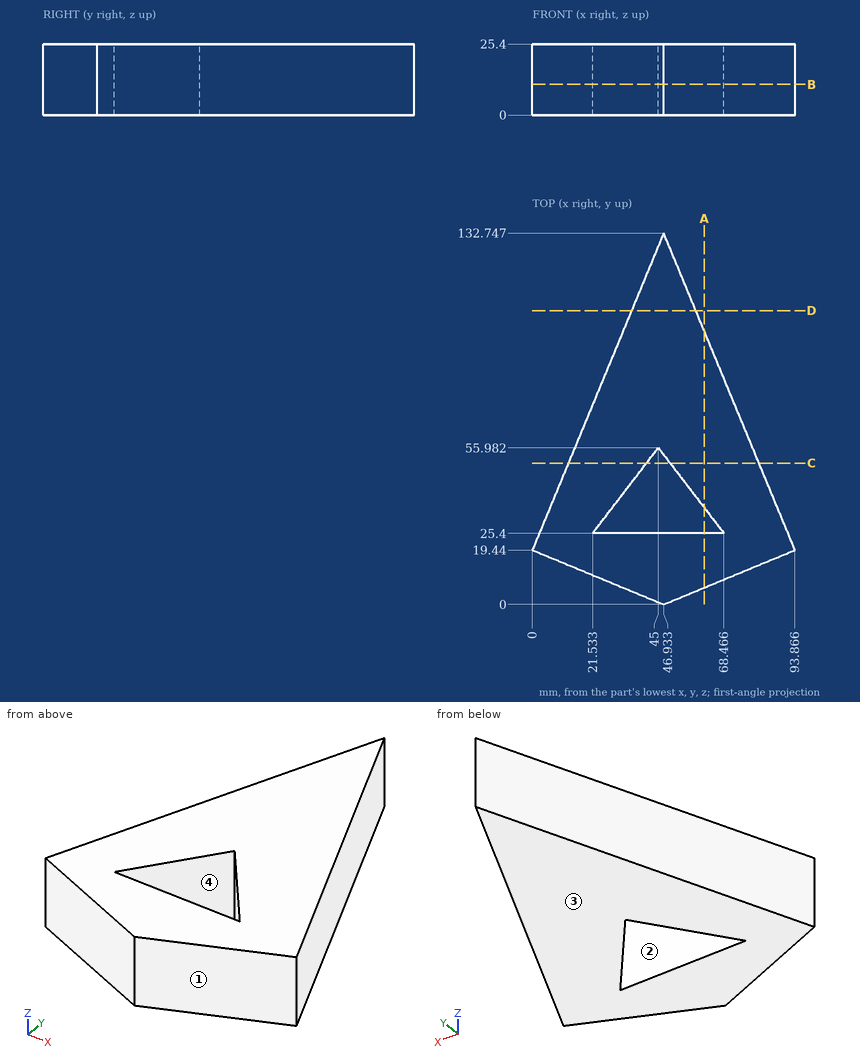
Geometry: see drawing. Coordinates: mm, zero at the bounding-box minimum. Coordinates: 2 decimals unless noted, no trailing zeros. Loops run counter-clockwise (first coordinate to the right, second up) from the corner with the lowest first, then second, coordinate; pieces in that order, holes last. Notation, with made-up numbers: M -40,64 L -20,64 A23 ccw -20,101 Z; hole C 16.5,48 d4. An arc over 180 degrees is marked long. Answer in a Markdown table with one row per item.
Q1. Draft query along Y for the marked faces 1, 2, 3 and 4. Return one class per face: pulls with the +Y half, pulls with the -Y half, needs draft (parallel to the pull), parting line crosses it, or undercut.
Answers below:
| item | result |
|---|---|
| face 1 | pulls with the -Y half |
| face 2 | undercut |
| face 3 | needs draft |
| face 4 | undercut |
Q2. First-contact query: pin 1 (2 mm diameter, centred on y = 32, z = 21.5, fed in from +X); pin 2 (8 mm diameter, centred on x = 69, z = 12.5, fed in from -Y); pin 3 (7.5 mm diameter, centred on x = 51, z = 10.5, fed in from +Y). Flat tips, straight axial feed; report the tip coordinate or a pass-through.
Answers below:
| item | result |
|---|---|
| pin 1 | stops at x = 89.08 |
| pin 2 | stops at y = 7.48 |
| pin 3 | stops at y = 131.98 |
Q3. Section B-B on z = 11. Return the cut outline in (x, y), plus the area to 3 significant figures.
Answers below:
| item | result |
|---|---|
| outline | M 0,19.44 L 46.93,0 L 93.87,19.44 L 46.93,132.75 Z; hole M 21.53,25.4 L 68.47,25.4 L 45,55.98 Z |
| area | 5,510 mm^2 |
Q4. Section D-D on y = 105. Return the cut outline in (x, z).
Answers below:
| item | result |
|---|---|
| outline | M 35.44,0 L 58.43,0 L 58.43,25.4 L 35.44,25.4 Z |
Q5. Section A-A on x = 61.5. Return the cut outline in (y, z).
Answers below:
| item | result |
|---|---|
| outline | M 6.03,0 L 25.4,0 L 25.4,25.4 L 6.03,25.4 Z; M 34.48,0 L 97.58,0 L 97.58,25.4 L 34.48,25.4 Z |
Q6. Section C-C on y = 50.5. Return the cut outline in (x, z) (1 decimal).
Answers below:
| item | result |
|---|---|
| outline | M 12.9,0 L 40.8,0 L 40.8,25.4 L 12.9,25.4 Z; M 49.2,0 L 81,0 L 81,25.4 L 49.2,25.4 Z |
Q7. Ray query, probe 1 along Y at (x, z) = (41, 9) (1 decimal); probe 2 along X at (y, z) = (41.5, 12.25); probe 3 along Y at (x, z) = (67, 9.75) (1 decimal). Return the intervals inside material, ascending. Write a range as from..to.
Answers below:
| item | result |
|---|---|
| probe 1 | y = 2.5..25.4, 50.8..118.4 |
| probe 2 | x = 9.14..33.89, 56.11..84.73 |
| probe 3 | y = 8.3..25.4, 27.3..84.3 |
